Verification items for the finished model (mm, model axes). Give positions to 0.01 mm unless a question says otherwise; leave off trailing zeros. Order: outer loops, then holes, each group sorted by start corner. A loop starts at its lowest first (then second) coordinate and runs counter-clockwise, first axis right, second up. Notation, with made-up numbers: (52.25, 10.5) - (75.25, 10.5) arc R25 cw to (75.25, 35.5) - close; hole circle Ø11 at (56, -17). An arc over 180 degrees is marked (long way). Answer as a JSON object with one key per item and string values.
```python
from build123d import *

# Parameters (mm, degrees)
SKETCH1_W           = 10
SKETCH1_H           = 55
SKETCH1_R           = 1.2
SKETCH1_R_2         = 2.75
BOSS_EXTRUDE1_DEPTH = 4
FILLET1_R           = 1


with BuildPart() as part:
    # Sketch1 → Boss-Extrude1 (new body)
    with BuildSketch(Plane.XY):
        with Locations((5, 27.5)):
            Rectangle(SKETCH1_W, SKETCH1_H)
        with Locations((7.4, 5)):
            Circle(SKETCH1_R, mode=Mode.SUBTRACT)
        with Locations((7.4, 14.9)):
            Circle(SKETCH1_R, mode=Mode.SUBTRACT)
        with Locations((5, 43.792878619)):
            Circle(SKETCH1_R_2, mode=Mode.SUBTRACT)
    extrude(amount=BOSS_EXTRUDE1_DEPTH)

    # Fillet1
    fillet1_edges = [part.edges().sort_by_distance(p)[0] for p in [
        (10, 27.5, 4),
        (5, 55, 4),
        (0, 27.5, 4),
        (5, 55, 0),
        (10, 27.5, 0),
        (5, 0, 0),
        (0, 27.5, 0),
        (0, 55, 2),
        (10, 55, 2),
        (10, 0, 2),
        (0, 0, 2),
        (5, 0, 4),
    ]]
    fillet(fillet1_edges, radius=FILLET1_R)


solid = part.part
```
(1) Section check D-D (y = 21). Record the cut outline in (x, z), then the cut area to 3 significant figures.
Computed values:
{"outline": "(0, 1) arc R1 ccw to (1, 0) - (9, 0) arc R1 ccw to (10, 1) - (10, 3) arc R1 ccw to (9, 4) - (1, 4) arc R1 ccw to (0, 3) - close", "area": "39.1 mm²"}
(2) Release check for a two-part mould opening along Y. For faces 1 (the flat face through (10, 27, 2)), 2 (the cylindrical face through (5.056, 0.285, 0.301)), 3 (the cylindrical face through (6.269, 41.353, 1.972)) record: pulls with the +Y half, pulls with the -Y half, needs draft (parallel to the pull), parting line crosses it, or undercut.
Computed values:
{"face 1": "needs draft", "face 2": "pulls with the -Y half", "face 3": "undercut"}
(3) Section check B-B (x = 5). Record the cut outline in (y, z).
Computed values:
{"outline": "(0, 1) arc R1 ccw to (1, 0) - (41.04, 0) - (41.04, 4) - (1, 4) arc R1 ccw to (0, 3) - close; (46.54, 0) - (54, 0) arc R1 ccw to (55, 1) - (55, 3) arc R1 ccw to (54, 4) - (46.54, 4) - close"}
(4) Gauge pin test, flat end, axial feed: pin 1 Ø3 at (x, y) = (7, 37) entering from -Z. Record the tip position at first contact, or that the pin passes through.
Computed values:
{"pin 1": "stops at z = 0"}
(5) Section check C-C (z = 1.6). Record the cut outline in (x, y), then the cut area to 3 significant figures.
Computed values:
{"outline": "(0, 1) arc R1 ccw to (1, 0) - (9, 0) arc R1 ccw to (10, 1) - (10, 54) arc R1 ccw to (9, 55) - (1, 55) arc R1 ccw to (0, 54) - close; hole circle Ø5.5 at (5, 43.79); hole circle Ø2.4 at (7.4, 5); hole circle Ø2.4 at (7.4, 14.9)", "area": "516 mm²"}
(6) Section check A-A (y = 5). Record the cut outline in (x, z), then the cut area to 3 significant figures.
Computed values:
{"outline": "(0, 1) arc R1 ccw to (1, 0) - (6.2, 0) - (6.2, 4) - (1, 4) arc R1 ccw to (0, 3) - close; (8.6, 0) - (9, 0) arc R1 ccw to (10, 1) - (10, 3) arc R1 ccw to (9, 4) - (8.6, 4) - close", "area": "29.5 mm²"}
(7) Material ranges on line 1 along Y through (x, z) = (7.4, 2.65); line 2 along Y through (x, z) = (8.25, 3.2); line 3 along Y through (x, z) = (5, 1.3), recorded low to high. Write a range as [from, to].
Computed values:
{"line 1": "y = [0, 3.8], [6.2, 13.7], [16.1, 42.45], [45.14, 55]", "line 2": "y = [0.02, 4.15], [5.85, 14.05], [15.75, 54.98]", "line 3": "y = [0, 41.04], [46.54, 55]"}
